Build history of the part. All positions in model axes, mm. Face numbers are marked on the shaded views. A direction names the side the tool comes from. Round coordinates to 2 decimals unless told otherwise and drop trailing zeros. Loops run counter-clockwise (first coordinate to the right, second up) from the corner with the lowest first, then second, coordinate; pieces in that order, holes last. Notation, with made-up numbers: (60.25, 51.5) - (110.25, 51.5) arc R7 cw to (110.25, 61.5) - close; hole circle Ø11 at (60.25, -10.5). An arc over 180 degrees is marked (long way). One line per question, with ' | ' between items. Start each with the question number.
from build123d import *

# Parameters (mm, degrees)
SKETCH1_R           = 5.5
BOSS_EXTRUDE1_DEPTH = 6
CUT_EXTRUDE1_START  = 6
CUT_EXTRUDE1_DEPTH  = 5.4
SKETCH3_R           = 0.791791972
CUT_EXTRUDE2_DEPTH  = 6
CHAMFER1_SIZE       = 0.6


with BuildPart() as part:
    # Sketch1 → Boss-Extrude1 (new body)
    with BuildSketch(Plane(origin=(0, 0, 0), x_dir=(1, 0, 0), z_dir=(0, 1, 0))):
        Circle(SKETCH1_R)
    extrude(amount=BOSS_EXTRUDE1_DEPTH)

    # Sketch2 → Cut-Extrude1 (cut)
    with BuildSketch(Plane(origin=(0, 0, 0), x_dir=(1, 0, 0), z_dir=(0, 1, 0)).offset(CUT_EXTRUDE1_START)):
        Polygon((4, -2.309401077), (4, 2.309401077), (0, 4.618802154), (-4, 2.309401077), (-4, -2.309401077), (0, -4.618802154), align=None)
    extrude(amount=-CUT_EXTRUDE1_DEPTH, mode=Mode.SUBTRACT)

    # Sketch3 → Cut-Extrude2 (cut)
    with BuildSketch(Plane(origin=(0, 0, 0), x_dir=(1, 0, 0), z_dir=(0, 1, 0))):
        with Locations((-5.5, 0)):
            Circle(SKETCH3_R)
        with Locations((-2.75, 4.763139721)):
            Circle(SKETCH3_R)
        with Locations((2.75, 4.763139721)):
            Circle(SKETCH3_R)
        with Locations((5.5, 0)):
            Circle(SKETCH3_R)
        with Locations((2.75, -4.763139721)):
            Circle(SKETCH3_R)
        with Locations((-2.75, -4.763139721)):
            Circle(SKETCH3_R)
    extrude(amount=CUT_EXTRUDE2_DEPTH, mode=Mode.SUBTRACT)

    # Chamfer1
    chamfer1_edges = [part.edges().sort_by_distance(p)[0] for p in [
        (4.763139721, 0, 2.75),
        (4.763139721, 0, -2.75),
        (0, 0, -5.5),
        (-4.763139721, 0, -2.75),
        (-4.763139721, 0, 2.75),
        (0, 0, 5.5),
        (-2.354104014, 0, -4.077427759),
        (2.354104014, 0, -4.077427759),
        (-4.708208028, 0, 0),
        (-2.354104014, 0, 4.077427759),
        (2.354104014, 0, 4.077427759),
        (4.708208028, 0, 0),
    ]]
    chamfer(chamfer1_edges, length=CHAMFER1_SIZE)


solid = part.part
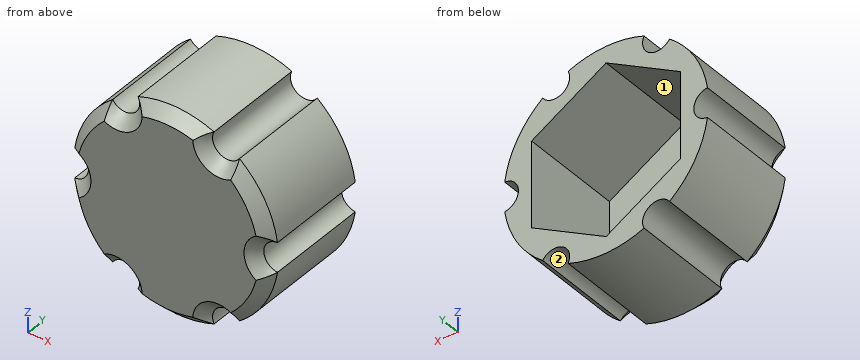
1) Saw through at A-A on y = 3. Write the cut outline in (x, z).
2) Tool access for the marked faces 1 and 2: list every direction of +Z, -Z, +X, -X, +Y, -Y with a clear straight run to the whole face (end or side of a thin tool).
3) Drop flat-ended pins along their axis: pin 1 (3.5 mm diameter, centred on y = 4, z = 0, fed in from -X); pin 2 (1 mm diameter, centred on x = -2.5, y = 2.5, fed in from -Z); pin 3 (1.5 mm diameter, centred on x = -3, z = -1.5, fed in from +Y). Give the stop position or say it passes through.
4) Wall check: line 1 (X direction, y = 1, z = 2.5); line 2 (X direction, y = 2.25, z = 3); line 3 (Y direction, x = 3.75, z = 0.75). Give the ranges that are in metal, low to high. Write a range as [from, to].
Answer key:
1) outline: (-5.44, -0.79) arc R5.5 ccw to (-3.41, -4.32) arc R0.79 cw to (-2.04, -5.11) arc R5.5 ccw to (2.04, -5.11) arc R0.79 cw to (3.41, -4.32) arc R5.5 ccw to (5.44, -0.79) arc R0.79 cw to (5.44, 0.79) arc R5.5 ccw to (3.41, 4.32) arc R0.79 cw to (2.04, 5.11) arc R5.5 ccw to (-2.04, 5.11) arc R0.79 cw to (-3.41, 4.32) arc R5.5 ccw to (-5.44, 0.79) arc R0.79 cw to start; hole (-4, -2.31) - (0, -4.62) - (4, -2.31) - (4, 2.31) - (0, 4.62) - (-4, 2.31) - close
2) face 1: +Y | face 2: +Y, -Y
3) pin 1: x = -5.44 | pin 2: z = -5.12 | pin 3: y = 0.6
4) line 1: [-4.9, -3.67], [3.67, 4.9] | line 2: [-4.61, -2.8], [2.8, 4.61] | line 3: [0, 0.6]
